Can you work these out from the model? Positions are in its coordinate system, mm. Coordinates: 2 decimals unless noted, no trailing zeros. Loops run counter-clockwise (first coordinate to the right, second up) from the corner with the lowest first, then second, coordinate; pieces in that order, holes last.
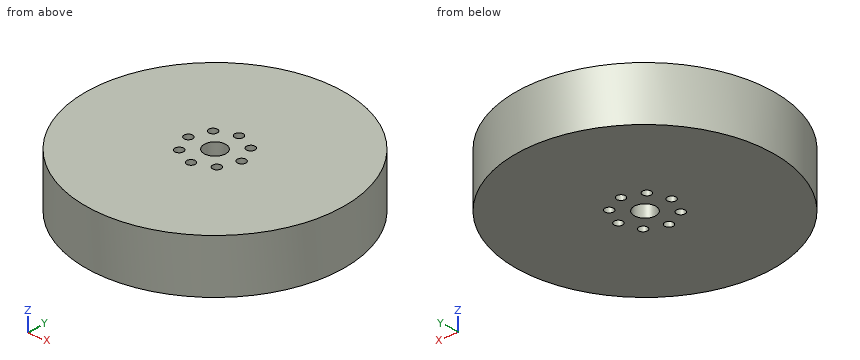
```python
from build123d import *

# Parameters (mm, degrees)
SKETCH1_R           = 48
BOSS_EXTRUDE1_DEPTH = 20
CUT_EXTRUDE1_REACH  = 72.767
SKETCH2_R           = 4
SKETCH2_R_2         = 1.6


with BuildPart() as part:
    # Sketch1 → Boss-Extrude1 (new body)
    with BuildSketch(Plane.XY):
        Circle(SKETCH1_R)
    extrude(amount=BOSS_EXTRUDE1_DEPTH)

    # Sketch2 → Cut-Extrude1 (cut, up to next)
    with BuildSketch(Plane(origin=(0, 0, 0), x_dir=(-1, 0, 0), z_dir=(0, 0, -1)), mode=Mode.PRIVATE) as cut_extrude1_sk1:
        Circle(SKETCH2_R)
    cut_extrude1_tool1 = extrude(cut_extrude1_sk1.sketch, amount=-CUT_EXTRUDE1_REACH, mode=Mode.PRIVATE) & part.part
    # Sketch2 → Cut-Extrude1 (cut, up to next)
    with BuildSketch(Plane(origin=(0, 0, 0), x_dir=(-1, 0, 0), z_dir=(0, 0, -1)), mode=Mode.PRIVATE) as cut_extrude1_sk2:
        with Locations((0, 10)):
            Circle(SKETCH2_R_2)
    cut_extrude1_tool2 = extrude(cut_extrude1_sk2.sketch, amount=-CUT_EXTRUDE1_REACH, mode=Mode.PRIVATE) & part.part
    # Sketch2 → Cut-Extrude1 (cut, up to next)
    with BuildSketch(Plane(origin=(0, 0, 0), x_dir=(-1, 0, 0), z_dir=(0, 0, -1)), mode=Mode.PRIVATE) as cut_extrude1_sk3:
        with Locations((7.071067812, 7.071067812)):
            Circle(SKETCH2_R_2)
    cut_extrude1_tool3 = extrude(cut_extrude1_sk3.sketch, amount=-CUT_EXTRUDE1_REACH, mode=Mode.PRIVATE) & part.part
    # Sketch2 → Cut-Extrude1 (cut, up to next)
    with BuildSketch(Plane(origin=(0, 0, 0), x_dir=(-1, 0, 0), z_dir=(0, 0, -1)), mode=Mode.PRIVATE) as cut_extrude1_sk4:
        with Locations((10, 0)):
            Circle(SKETCH2_R_2)
    cut_extrude1_tool4 = extrude(cut_extrude1_sk4.sketch, amount=-CUT_EXTRUDE1_REACH, mode=Mode.PRIVATE) & part.part
    # Sketch2 → Cut-Extrude1 (cut, up to next)
    with BuildSketch(Plane(origin=(0, 0, 0), x_dir=(-1, 0, 0), z_dir=(0, 0, -1)), mode=Mode.PRIVATE) as cut_extrude1_sk5:
        with Locations((7.071067812, -7.071067812)):
            Circle(SKETCH2_R_2)
    cut_extrude1_tool5 = extrude(cut_extrude1_sk5.sketch, amount=-CUT_EXTRUDE1_REACH, mode=Mode.PRIVATE) & part.part
    # Sketch2 → Cut-Extrude1 (cut, up to next)
    with BuildSketch(Plane(origin=(0, 0, 0), x_dir=(-1, 0, 0), z_dir=(0, 0, -1)), mode=Mode.PRIVATE) as cut_extrude1_sk6:
        with Locations((0, -10)):
            Circle(SKETCH2_R_2)
    cut_extrude1_tool6 = extrude(cut_extrude1_sk6.sketch, amount=-CUT_EXTRUDE1_REACH, mode=Mode.PRIVATE) & part.part
    # Sketch2 → Cut-Extrude1 (cut, up to next)
    with BuildSketch(Plane(origin=(0, 0, 0), x_dir=(-1, 0, 0), z_dir=(0, 0, -1)), mode=Mode.PRIVATE) as cut_extrude1_sk7:
        with Locations((-7.071067812, -7.071067812)):
            Circle(SKETCH2_R_2)
    cut_extrude1_tool7 = extrude(cut_extrude1_sk7.sketch, amount=-CUT_EXTRUDE1_REACH, mode=Mode.PRIVATE) & part.part
    # Sketch2 → Cut-Extrude1 (cut, up to next)
    with BuildSketch(Plane(origin=(0, 0, 0), x_dir=(-1, 0, 0), z_dir=(0, 0, -1)), mode=Mode.PRIVATE) as cut_extrude1_sk8:
        with Locations((-10, 0)):
            Circle(SKETCH2_R_2)
    cut_extrude1_tool8 = extrude(cut_extrude1_sk8.sketch, amount=-CUT_EXTRUDE1_REACH, mode=Mode.PRIVATE) & part.part
    # Sketch2 → Cut-Extrude1 (cut, up to next)
    with BuildSketch(Plane(origin=(0, 0, 0), x_dir=(-1, 0, 0), z_dir=(0, 0, -1)), mode=Mode.PRIVATE) as cut_extrude1_sk9:
        with Locations((-7.071067812, 7.071067812)):
            Circle(SKETCH2_R_2)
    cut_extrude1_tool9 = extrude(cut_extrude1_sk9.sketch, amount=-CUT_EXTRUDE1_REACH, mode=Mode.PRIVATE) & part.part
    add(cut_extrude1_tool1.solids().sort_by_distance((0, 0, 0))[0], mode=Mode.SUBTRACT)
    add(cut_extrude1_tool2.solids().sort_by_distance((0, 10, 0))[0], mode=Mode.SUBTRACT)
    add(cut_extrude1_tool3.solids().sort_by_distance((-7.071068, 7.071068, 0))[0], mode=Mode.SUBTRACT)
    add(cut_extrude1_tool4.solids().sort_by_distance((-10, 0, 0))[0], mode=Mode.SUBTRACT)
    add(cut_extrude1_tool5.solids().sort_by_distance((-7.071068, -7.071068, 0))[0], mode=Mode.SUBTRACT)
    add(cut_extrude1_tool6.solids().sort_by_distance((0, -10, 0))[0], mode=Mode.SUBTRACT)
    add(cut_extrude1_tool7.solids().sort_by_distance((7.071068, -7.071068, 0))[0], mode=Mode.SUBTRACT)
    add(cut_extrude1_tool8.solids().sort_by_distance((10, 0, 0))[0], mode=Mode.SUBTRACT)
    add(cut_extrude1_tool9.solids().sort_by_distance((7.071068, 7.071068, 0))[0], mode=Mode.SUBTRACT)


solid = part.part
```
(1) I'm going to push flat-ended pins straight in: pin 1 (1.9 mm diameter, centred on x = 0, y = 10, fed in from +Z); pin 2 (1 mm diameter, centred on y = 16.5, z = 10.5, fed in from -X); pin 3 (12 mm diameter, centred on y = 21, z = 4.5, fed in from +X); pin 4 (10 mm diameter, centred on y = -3, z = 13, fed in from -X). Where does each tip first touch, or does it pass through?
Check values:
pin 1: passes through
pin 2: stops at x = -45.25
pin 3: stops at x = 45.6
pin 4: stops at x = -48
(2) I want a section at D-D on z = 6.5. State how many separate pieces and enclosed holes the cut face has, then the cut area to 3 significant figures.
Check values:
separate pieces: 1
enclosed holes: 9
area: 7,120 mm2
(3) I want a section at B-B on y = -10. Write out the boundary of the cut face in (x, z).
Check values:
outline: (-46.95, 0) - (-1.6, 0) - (-1.6, 20) - (-46.95, 20) - close; (1.6, 0) - (46.95, 0) - (46.95, 20) - (1.6, 20) - close
(4) I want a section at A-A on x = 0. Write out the boundary of the cut face in (y, z).
Check values:
outline: (-48, 0) - (-11.6, 0) - (-11.6, 20) - (-48, 20) - close; (-8.4, 0) - (-4, 0) - (-4, 20) - (-8.4, 20) - close; (4, 0) - (8.4, 0) - (8.4, 20) - (4, 20) - close; (11.6, 0) - (48, 0) - (48, 20) - (11.6, 20) - close
(5) If I drill on probe 1 along Y at (x, z) = (0, 9.5); probe 2 along X at (y, z) = (7, 16); probe 3 along X at (y, z) = (-8, 13.5), over which ranges is the centre line in solid material (lowest first)?
Check values:
probe 1: y = -48 to -11.6, -8.4 to -4, 4 to 8.4, 11.6 to 48
probe 2: x = -47.49 to -8.67, -5.47 to 5.47, 8.67 to 47.49
probe 3: x = -47.33 to -8.37, -5.77 to 5.77, 8.37 to 47.33
